Geometry: final body of the model. Coordinates: model frame, mm. A direction names the side the tool comes from. Round coordinates to 2 decimals unless told otherwise and drop trailing zeros. Loops run counter-clockwise (first coordinate to the right, second up) from the corner with the lowest first, then second, coordinate; pieces in that order, holes last. Notation, with made-up numbers: (-4, 23.5) - (33, 23.5) arc R6 cw to (33, 34.5) - close; hole circle Ø5 at (-20, -19.75). An arc over 180 degrees is marked (long way). Answer as CSV lines item,"result".
from build123d import *

# Parameters (mm, degrees)
SKETCH1_W           = 112.5
SKETCH1_H           = 238
BOSS_EXTRUDE1_DEPTH = 6
SKETCH2_R           = 30.970562748
SKETCH2_R_2         = 10
SKETCH2_R_3         = 1.4
SKETCH2_R_4         = 1.75
BOSS_EXTRUDE2_DEPTH = 6
SKETCH3_W           = 112.5
SKETCH3_H           = 238
CUT_EXTRUDE1_DEPTH  = 6


with BuildPart() as part:
    # Sketch1 → Boss-Extrude1 (new body)
    with BuildSketch(Plane(origin=(0, 0, 0), x_dir=(0, 0, -1), z_dir=(1, 0, 0))):
        Rectangle(SKETCH1_W, SKETCH1_H)
    extrude(amount=BOSS_EXTRUDE1_DEPTH)

    # Sketch2 → Boss-Extrude2 (add)
    with BuildSketch(Plane(origin=(6, 0, 0), x_dir=(0, 0, -1), z_dir=(1, 0, 0))):
        with Locations((0, -82.029437252)):
            Circle(SKETCH2_R)
        with Locations((0, -99)):
            Circle(SKETCH2_R_2, mode=Mode.SUBTRACT)
        with Locations((-4.5, -60.558874503)):
            Circle(SKETCH2_R_3, mode=Mode.SUBTRACT)
        with Locations((0, -60.558874503)):
            Circle(SKETCH2_R_3, mode=Mode.SUBTRACT)
        with Locations((4.5, -60.558874503)):
            Circle(SKETCH2_R_3, mode=Mode.SUBTRACT)
        with Locations((0, -65.058874503)):
            Circle(SKETCH2_R_3, mode=Mode.SUBTRACT)
        with Locations((4.5, -65.058874503)):
            Circle(SKETCH2_R_3, mode=Mode.SUBTRACT)
        with Locations((0, -69.558874503)):
            Circle(SKETCH2_R_3, mode=Mode.SUBTRACT)
        with Locations((4.5, -69.558874503)):
            Circle(SKETCH2_R_3, mode=Mode.SUBTRACT)
        with Locations((-4.5, -65.058874503)):
            Circle(SKETCH2_R_3, mode=Mode.SUBTRACT)
        with Locations((-4.5, -69.558874503)):
            Circle(SKETCH2_R_3, mode=Mode.SUBTRACT)
        with Locations((0, -82.029437252)):
            Circle(SKETCH2_R_4, mode=Mode.SUBTRACT)
        with BuildLine():
            Line((-14.320562748, -74.029437252), (-14.320562748, -90.029437252))
            ThreePointArc((-14.320562748, -90.029437252), (-16.970562748, -92.679437252), (-19.620562748, -90.029437252))
            Line((-19.620562748, -90.029437252), (-19.620562748, -74.029437252))
            ThreePointArc((-19.620562748, -74.029437252), (-16.970562748, -71.379437252), (-14.320562748, -74.029437252))
        make_face(mode=Mode.SUBTRACT)
    extrude(amount=BOSS_EXTRUDE2_DEPTH)

    # Sketch3 → Cut-Extrude1 (cut)
    with BuildSketch(Plane.ZY):
        Rectangle(SKETCH3_W, SKETCH3_H)
    extrude(amount=-CUT_EXTRUDE1_DEPTH, mode=Mode.SUBTRACT)


solid = part.part
(1) Section B-B (y = -101). Output: boundary loops of the cut face in (x, z).
Findings below:
outline,"(6, -24.48) - (12, -24.48) - (12, -9.8) - (6, -9.8) - close; (6, 9.8) - (12, 9.8) - (12, 24.48) - (6, 24.48) - close"
(2) Section A-A (z = 0). Output: boundary loops of the cut face in (x, y).
Findings below:
outline,"(6, -113) - (12, -113) - (12, -109) - (6, -109) - close; (6, -89) - (12, -89) - (12, -83.78) - (6, -83.78) - close; (6, -80.28) - (12, -80.28) - (12, -70.96) - (6, -70.96) - close; (6, -68.16) - (12, -68.16) - (12, -66.46) - (6, -66.46) - close; (6, -63.66) - (12, -63.66) - (12, -61.96) - (6, -61.96) - close; (6, -59.16) - (12, -59.16) - (12, -51.06) - (6, -51.06) - close"
(3) Material intervals for line 1 along Z through (x, y) = (9.05, -81); line 2 along Z through (x, y) = (11.3, -81.5); line 3 along Y through (x, z) = (8.25, 4), sorted ascending.
Findings below:
line 1,"-30.95 to -1.42, 1.42 to 14.32, 19.62 to 30.95"
line 2,"-30.97 to -1.67, 1.67 to 14.32, 19.62 to 30.97"
line 3,"-112.74 to -108.17, -89.83 to -70.87, -68.25 to -66.37, -63.75 to -61.87, -59.25 to -51.32"
(4) Section D-D (x = 8.4). Give the number of separate pieces and of enclosed holes in the cut face, and give its area (3 significant figures).
Findings below:
separate pieces,"1"
enclosed holes,"12"
area,"2,530 mm2"
(5) Access query for faces 5 (the face through (6, -82, 6)), 6 (the face through (9, -82, 14.321)). Directions: +Z, -Z, +X, -X, +Y, -Y. A direction counts if a zero-diameter tool reaches every point of the face in a straight line with its end or side. Return the directions, or none.
Findings below:
face 5,"+Z, -Z, -X, +Y, -Y"
face 6,"+X, -X"
(6) Pin query (flat end, axial travel): P1, Ø2, axis at x = 7, y = -68, coming from the +Z side; P2, Ø1.5, axis at x = 7.5, z = -19, coming from the -Y side; P3, Ø2, axis at x = 9.5, y = -104.5, coming from the +Z side. Return the tip coordinate at first contact, or that it passes through.
Findings below:
P1,"z = 28.1"
P2,"y = -107.05"
P3,"z = 22.32"
(7) Section C-C (z = 8). Output: boundary loops of the cut face in (x, y).
Findings below:
outline,"(6, -111.95) - (12, -111.95) - (12, -105) - (6, -105) - close; (6, -93) - (12, -93) - (12, -52.11) - (6, -52.11) - close"
(8) Draft query along Z for faces 1 (the face through (9, -109.5, -14.3)), 2 (the face through (8.958, -83.738, 0.379)), 3 (the face through (8.96, -63.67, 0.18)), 4 (the face through (12, -82, -6)). Return one class per face: pulls with the +Z half, pulls with the -Z half, needs draft (parallel to the pull), parting line crosses it, or undercut.
Findings below:
face 1,"parting line crosses it"
face 2,"undercut"
face 3,"undercut"
face 4,"needs draft"
